from build123d import *

# Parameters (mm, degrees)
F0_R     = 6
F1_DEPTH = 10
F2_W     = 60
F2_H     = 35
F3_DEPTH = 50
F4_R     = 12
F5_SIZE2 = 5
F5_SIZE  = 5
F7_DEPTH = 60.001


with BuildPart() as f1:
    # F0 (on Top) → F1 (new body)
    with BuildSketch(Plane.XY):
        with BuildLine():
            Line((60, 17.5), (-60, 17.5))
            ThreePointArc((-60, 17.5), (-77.5, 0), (-60, -17.5))
            Line((-60, -17.5), (60, -17.5))
            ThreePointArc((60, -17.5), (77.5, 0), (60, 17.5))
        make_face()
        with Locations((-60, 0)):
            Circle(F0_R, mode=Mode.SUBTRACT)
        with Locations((60, 0)):
            Circle(F0_R, mode=Mode.SUBTRACT)
    extrude(amount=F1_DEPTH)

    # F2 (on face) → F3 (join)
    with BuildSketch(Plane.XY.offset(10)):
        Rectangle(F2_W, F2_H)
    extrude(amount=F3_DEPTH)

    # F4
    f4_edges = [f1.edges().sort_by_distance(p)[0] for p in [
        (30, 0, 10),
        (-30, 0, 10),
    ]]
    fillet(f4_edges, radius=F4_R)

    # F5
    f5_edges = [f1.edges().sort_by_distance(p)[0] for p in [
        (30, 0, 60),
        (-30, 0, 60),
    ]]
    chamfer(f5_edges, length=F5_SIZE, length2=F5_SIZE2)

    # F6 (on face) → F7 (cut, through all)
    with BuildSketch(Plane.XY.offset(60)):
        Polygon((-9, -7.5), (-9, -17.5), (9, -17.5), (9, -7.5), (15, -7.5), (15, 2.5), (-15, 2.5), (-15, -7.5), align=None)
    extrude(amount=-F7_DEPTH, mode=Mode.SUBTRACT)


solid = f1.part
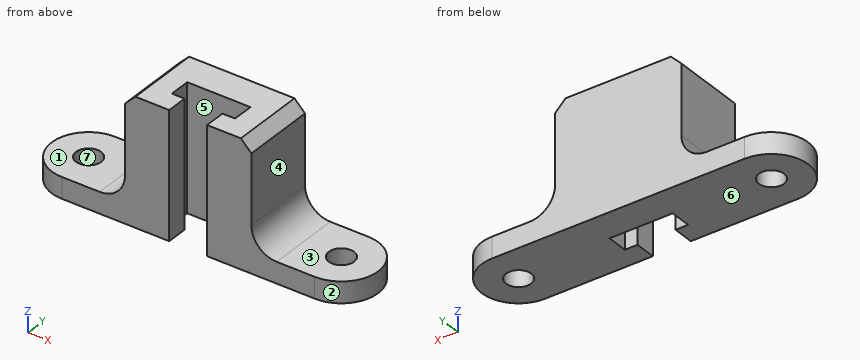
Part model, mm, in its own coordinate system. Face numbers are marked on the shaded views. A direction names the side the tool comes from. Coordinates: 2 decimals unless noted, no trailing zeros. Loops run counter-clockwise (first coordinate to the right, second up) from the corner with the lowest first, then second, coordinate; pieces in that order, holes last. Notation, with made-up numbers: (46.5, 2.5) -> (100.5, 2.5) arc R23 ccw to (100.5, 10.5) -> close; hole circle Ø5 at (14.25, 30.5). An arc over 180 degrees is marked (long way). Use a Markdown table: item, result. Add a question column.
Item 1: Pull direction X, two halves, no side cores. Call the marked faces 4, 5, 6 and 7: +X half, -X half, draft (parallel to the pull), parting line (faces both ways), or undercut.
Item 2: Band-saw the part on A-A on y = -14. Write the cut outline in (x, z).
Item 3: Flat gauge pins, fed straight in: P1, Ø8, axis at y = -2, z = 22.5, coming from the -X side; P2, Ø17.5, axis at x = -54, y = 6, coming from the +Z side; P3, Ø16.5, axis at y = 1, z = 38, coming from the +X side. Where does each tip first touch, or does it go through?
Item 4: Band-saw the part on D-D on z = 49. Write the cut outline in (x, y).
Item 5: Band-saw the part on B-B on z = 8. Write the cut outline in (x, y).
Item 6: Band-saw the part on C-C on y = 0. Write the cut outline in (x, z), plus the area to 3 significant figures.
Item 7: Which spindle directions (+Z, -Z, +X, -X, +Y, -Y) get a long thin tool onto all of the face, cutting with end or side? Do the marked faces 1, 2 and 3. Say none if no direction does.
Item 8: Probe probe 1 along Y at (x, z) = (-60, 6.75); probe 2 along X at (y, z) = (-8, 51.5); probe 3 along X at (y, z) = (1, 47). List the from-to ranges inside material, lowest first.
Geometry says:
| question | item | result |
|---|---|---|
| 1 | face 4 | +X half |
| 1 | face 5 | undercut |
| 1 | face 6 | draft |
| 1 | face 7 | undercut |
| 2 | outline | (-70.5, 0) -> (-9, 0) -> (-9, 60) -> (-25, 60) -> (-30, 55) -> (-30, 22) arc R12 cw to (-42, 10) -> (-70.5, 10) -> close; (9, 0) -> (70.5, 0) -> (70.5, 10) -> (42, 10) arc R12 cw to (30, 22) -> (30, 55) -> (25, 60) -> (9, 60) -> close |
| 3 | P1 | x = -30.52 |
| 3 | P2 | z = 10 |
| 3 | P3 | x = 30 |
| 4 | outline | (-30, -17.5) -> (-9, -17.5) -> (-9, -7.5) -> (-15, -7.5) -> (-15, 2.5) -> (15, 2.5) -> (15, -7.5) -> (9, -7.5) -> (9, -17.5) -> (30, -17.5) -> (30, 17.5) -> (-30, 17.5) -> close |
| 5 | outline | (-60, -17.5) -> (-9, -17.5) -> (-9, -7.5) -> (-15, -7.5) -> (-15, 2.5) -> (15, 2.5) -> (15, -7.5) -> (9, -7.5) -> (9, -17.5) -> (60, -17.5) arc R17.5 ccw to (60, 17.5) -> (-60, 17.5) arc R17.5 ccw to start; hole circle Ø12 at (-60, 0); hole circle Ø12 at (60, 0) |
| 6 | outline | (-77.5, 0) -> (-66, 0) -> (-66, 10) -> (-77.5, 10) -> close; (-54, 0) -> (-15, 0) -> (-15, 60) -> (-25, 60) -> (-30, 55) -> (-30, 22) arc R12 cw to (-42, 10) -> (-54, 10) -> close; (15, 0) -> (54, 0) -> (54, 10) -> (42, 10) arc R12 cw to (30, 22) -> (30, 55) -> (25, 60) -> (15, 60) -> close; (66, 0) -> (77.5, 0) -> (77.5, 10) -> (66, 10) -> close |
| 6 | area | 2,550 mm² |
| 7 | face 1 | +Z, -X, +Y, -Y |
| 7 | face 2 | +Z, -Z, +X |
| 7 | face 3 | +Z, +X, +Y, -Y |
| 8 | probe 1 | -17.5 to -6, 6 to 17.5 |
| 8 | probe 2 | -30 to -9, 9 to 30 |
| 8 | probe 3 | -30 to -15, 15 to 30 |
